Input: part model. Units: mm. Frame: model coordinates. Face numbers are marked on the shaded views. Give positions to 0.01 mm unless a question says otherwise; leave off trailing zeros. Order: outer loops, then holes, each group sorted by start corner. A loop starts at its lowest first (then second) coordinate and runs counter-clockwise, first axis right, second up. Notation, with made-up numbers: (-36, 43) - (-2, 43) arc R19 ccw to (-2, 62) - close; hole circle Ø7 at (11, -37). An arc over 180 degrees is marked (long way). Answer in a Markdown table with one row per item. Add a question column.
1. Section query D-D on y = -15. Return loops of the section in (x, z).
2. Mould query, pull axis X, two halves, no side actions, for the marked faces 1 and 2. Classes: released by +X, released by -X, zero draft, split by the parting line, or undercut.
3. Section query B-B on x = 0. Return loops of the section in (y, z), and give its area (3 significant figures).
4. Ray query, line 1 (X direction, y = -60, z = 0); line 2 (Y direction, x = -3, z = -0.25); line 3 (Z direction, x = 0.25, y = -4.5). Return the intervals inside material, ascending. Write a range as [from, to].
5. Contact query for flat-ended pins moving along their axis: pin 1 (3 mm diameter, centred on x = 2.5, y = -56.5, fed in from +Z); pin 2 (3.5 mm diameter, centred on x = 0, z = -1.5, fed in from -Y). Output: stop coordinate, or through.
6. Section query C-C on y = -54. Return loops of the section in (x, z), and give its area (3 significant figures).
7. Section query A-A on z = 0. Return loops of the section in (x, y).
```python
from build123d import *

# Parameters (mm, degrees)
SKETCH_1_R          = 5
EXTRUDE_1_DEPTH     = 7
EXTRUDE_START       = 68
SKETCH_2_R          = 5
EXTRUDE_2_DEPTH     = 68
SKETCH_3_R          = 3.5
CUT_EXTRUDE_1_DEPTH = 20


with BuildPart() as part:
    # ｽｹｯﾁ1 → ﾎﾞｽ - 押し出し1 (new body)
    with BuildSketch(Plane(origin=(0, 0, 0), x_dir=(1, 0, 0), z_dir=(0, 1, 0))):
        with Locations(Location((0, 0, 0), (0, 0, 270))):
            Circle(SKETCH_1_R)
    extrude(amount=EXTRUDE_1_DEPTH)

    # ｽｹｯﾁ2 → ﾎﾞｽ - 押し出し2 (add)
    with BuildSketch(Plane.XZ.offset(EXTRUDE_START)):
        with Locations(Location((0, 0, 0), (0, 0, 270))):
            Circle(SKETCH_2_R)
    extrude(amount=-EXTRUDE_2_DEPTH)

    # ｽｹｯﾁ3 → ｶｯﾄ - 押し出し1 (cut)
    with BuildSketch(Plane.XZ.offset(68)):
        with Locations(Location((0, 0, 0), (0, 0, 270))):
            Circle(SKETCH_3_R)
    extrude(amount=-CUT_EXTRUDE_1_DEPTH, mode=Mode.SUBTRACT)


solid = part.part
```
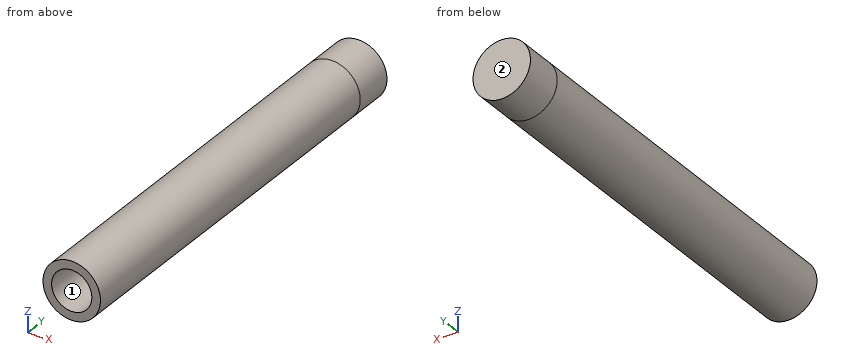
Answer:
| question | item | result |
|---|---|---|
| 1 | outline | circle Ø10 at (0, 0) |
| 2 | face 1 | undercut |
| 2 | face 2 | zero draft |
| 3 | outline | (-68, -5) - (7, -5) - (7, 5) - (-68, 5) - (-68, 3.5) - (-48, 3.5) - (-48, -3.5) - (-68, -3.5) - close |
| 3 | area | 610 mm² |
| 4 | line 1 | x = [-5, -3.5], [3.5, 5] |
| 4 | line 2 | y = [-48, 7] |
| 4 | line 3 | z = [-4.99, 4.99] |
| 5 | pin 1 | stops at z = 4.9 |
| 5 | pin 2 | stops at y = -48 |
| 6 | outline | circle Ø10 at (0, 0); hole circle Ø7 at (0, 0) |
| 6 | area | 40.1 mm² |
| 7 | outline | (-5, -68) - (-3.5, -68) - (-3.5, -48) - (3.5, -48) - (3.5, -68) - (5, -68) - (5, 7) - (-5, 7) - close |
